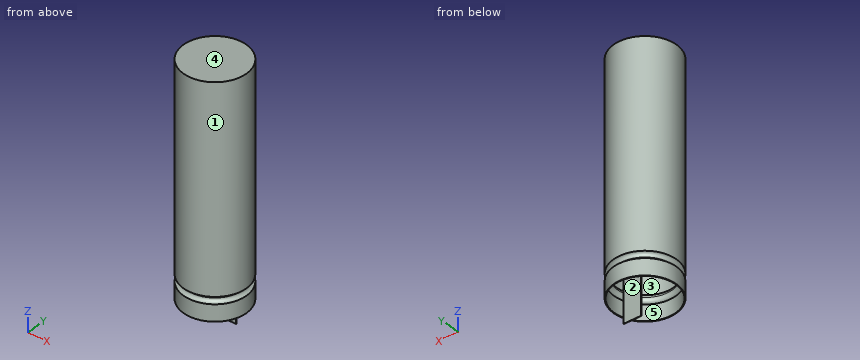
```python
from build123d import *

# Parameters (mm, degrees)
SKETCH_2_R      = 9
EXTRUDE_1_DEPTH = 32.5
SKETCH_3_R      = 1
SHELL_1_T       = -0.2
SKETCH_4_W      = 5
SKETCH_4_H      = 0.1
EXTRUDE_2_DEPTH = 73


with BuildPart() as part:
    # 草图2 → 凸台-拉伸1 (new, symmetric)
    with BuildSketch(Plane.XY):
        Circle(SKETCH_2_R)
    extrude(amount=EXTRUDE_1_DEPTH, both=True)

    # 草图3 → 切除-旋转1 (revolve, cut)
    with BuildSketch(Plane(origin=(0, 0, 0), x_dir=(1, 0, 0), z_dir=(0, 1, 0)), mode=Mode.PRIVATE) as cut_revolve_1_sk:
        with Locations((-9, 26.776971268)):
            Circle(SKETCH_3_R)
    revolve(cut_revolve_1_sk.sketch.rotate(Axis((0, 0, 0), (0, 0, -1)), 180), axis=Axis((0, 0, 0), (0, 0, -1)), mode=Mode.SUBTRACT)

    # 抽壳1
    shell_1_openings = [part.faces().sort_by_distance(p)[0] for p in [
        (0, 0, -32.5),
    ]]
    offset(amount=SHELL_1_T, openings=shell_1_openings, kind=Kind.INTERSECTION)

    # 草图4 → 凸台-拉伸2 (add)
    with BuildSketch(Plane(origin=(0, 0, 32.3), x_dir=(-1, 0, 0), z_dir=(0, 0, -1))):
        with Locations((0, 4.473785882)):
            Rectangle(SKETCH_4_W, SKETCH_4_H)
    extrude(amount=EXTRUDE_2_DEPTH)


solid = part.part
```
Input: part model. Units: mm. Frame: model coordinates. Face numbers are marked on the shaded views. A direction names the side the tool comes from. Coordinates: 2 decimals unless noted, no trailing zeros. Write each loop counter-clockwise with the first axis right and the second up, starting at its lowest first coordinate (ties: lowest second). Pieces come first, ordered by that corner, then holes. Notation, with made-up numbers: (-20.75, 17.5) - (5.25, 17.5) arc R32 ccw to (5.25, 48.5) - close; hole circle Ø4 at (64, 13.5). An arc over 180 degrees is marked (long way). Put each result on its own line as item: value. Start each with the question number.
1) Reachability of the marked faces 1 and 2 from +Z, -Z, +X, -X, +Y, -Y: full face, straight path, thin tool, end or side. Return the list, or none.
2) Mould query, pull axis Z, two halves, no side actions, for the marked faces 3, 4 and 5. Classes: pulls with the +Z half, pulls with the -Z half, needs draft (parallel to the pull), parting line crosses it, or undercut.
3) Cut plane B-B (y = 0). Return the cut outline in (x, z), plus the area to 3 significant figures.
4) Cut plane C-C (x = 0). Return the cut outline in (y, z), plus the area to 3 significant figures.
5) Ray query, L1, parallel to X at y = 0.5, z = -28; L2, parallel to Z at x = 4, y = -5.75; L3, parallel to X at y = 6.75, z = 12. Return the intervals inside material, ascending.
6) Cut plane A-A (z = -11). Return the cut outline in (x, y), plus the area to 3 significant figures.
7) Contact query for flat-ended pins moving along their axis: pin 1 (10 mm diameter, centred on x = -7, z = -16.5, fed in from +Y); pin 2 (3 mm diameter, centred on x = -4, z = 5.5, fed in from +Y); pin 3 (1.5 mm diameter, centred on x = 1.5, y = -1.5, fed in from -Z). Output: stop coordinate, or through.
8) Cut plane D-D (z = -34.5). Return the cut outline in (x, y).
Resolved:
1. face 1: +Z, -Z
1. face 2: -Z
2. face 3: undercut
2. face 4: pulls with the +Z half
2. face 5: needs draft
3. outline: (-9, -32.5) - (-8.8, -32.5) - (-8.8, -27.96) arc R1.2 ccw to (-8.8, -25.59) - (-8.8, 32.3) - (8.8, 32.3) - (8.8, -25.59) arc R1.2 ccw to (8.8, -27.96) - (8.8, -32.5) - (9, -32.5) - (9, -27.78) arc R1 cw to (9, -25.78) - (9, 32.5) - (-9, 32.5) - (-9, -25.78) arc R1 cw to (-9, -27.78) - close
3. area: 29.9 mm2
4. outline: (-9, -32.5) - (-8.8, -32.5) - (-8.8, -27.96) arc R1.2 ccw to (-8.8, -25.59) - (-8.8, 32.3) - (4.42, 32.3) - (4.42, -40.7) - (4.52, -40.7) - (4.52, 32.3) - (8.8, 32.3) - (8.8, -25.59) arc R1.2 ccw to (8.8, -27.96) - (8.8, -32.5) - (9, -32.5) - (9, -27.78) arc R1 cw to (9, -25.78) - (9, 32.5) - (-9, 32.5) - (-9, -25.78) arc R1 cw to (-9, -27.78) - close
4. area: 37.2 mm2
5. L1: x = -8.99 to -8.79, 8.79 to 8.99
5. L2: z = 32.3 to 32.5
5. L3: x = -5.95 to -5.65, 5.65 to 5.95
6. outline: circle Ø18 at (0, 0); (-2.5, 4.42) - (2.5, 4.42) - (2.5, 4.52) - (-2.5, 4.52) - close; hole circle Ø17.6 at (0, 0)
6. area: 11.7 mm2
7. pin 1: stops at y = 8.77
7. pin 2: stops at y = 8.65
7. pin 3: stops at z = 32.3
8. outline: (-2.5, 4.42) - (2.5, 4.42) - (2.5, 4.52) - (-2.5, 4.52) - close
